The model under review builds one solid part; all positions refer to its coordinate system, in mm. Coordinates: 2 decimals unless noted, no trailing zeros. Loops run counter-clockwise (first coordinate to the right, second up) from the corner with the lowest first, then second, coordinate; pieces in that order, holes last. Notation, with made-up numbers: M -20,17 L 39,17 A19 ccw 39,49 Z; hole C 25.25,-31.5 d4. An arc over 180 degrees is marked long. Use CSV: the item, a comma, the result in double quotes. Start each with the question number.
1. Add section B-B, the plane y = -1.5. Write out the cut boundary in (x, z) (3 decimals), then the cut area to 3 significant figures.
2. Add section C-C, the plane z = 4.75. Write out the cut boundary in (x, y).
3. For L1, parallel to X at y = -5.25, z = 7.5; L2, parallel to X at y = -0.25, z = 2.25; L3, parallel to X at y = -1.75, z = 7.5, list the stretches that pass through material, from the lowest coordinate up.
4. Add section D-D, the plane x = 9. Write out the cut boundary in (y, z).
5. Draft analysis for pull direction X (two halves, no side actions). For faces 1 (the cylindrical face through (-0.22, -5.14, 0.9)), 2 (the cylindrical face through (15.235, -3.042, 7.303)), 3 (the cylindrical face through (-17.6, -1.48, 13.29)), state which applies: +X half, -X half, draft (parallel to the pull), parting line (faces both ways), or undercut.
6. Clearance check with flat-ended pins moving along their axes: P1, Ø1, axis at y = -4.5, z = 1.5, coming from the +X side; P2, Ø3, axis at x = -13.5, z = 7.075, coming from the -Y side; P3, Ø2, axis at x = -14.5, y = -4.5, coming from the -Z side; P4, Ø1, axis at x = -4.5, y = -4, coming from the +Z side. State where each tip first meets the part, or that it passes through.
7. Add section A-A, the plane x = 13.5. Write out the cut boundary in (y, z) (3 decimals), then the cut area to 3 significant figures.
from build123d import *

# Parameters (mm, degrees)
ESBO_O1_W                = 37
ESBO_O1_H                = 6
RESSALTO_EXTRUS_O1_DEPTH = 14.15
ESBO_O2_R                = 3.96875
CORTE_EXTRUS_O1_DEPTH    = 25.051455257
ESBO_O3_R                = 1.75
CORTE_EXTRUS_O2_DEPTH    = 13
FILETE2_R                = 3
FILETE3_R                = 3


with BuildPart() as part:
    # Esboço1 → Ressalto-extrusão1 (new body)
    with BuildSketch(Plane.XY):
        with Locations((0, -3)):
            Rectangle(ESBO_O1_W, ESBO_O1_H)
    extrude(amount=RESSALTO_EXTRUS_O1_DEPTH)

    # Esboço2 → Corte-extrusão1 (cut, through all)
    with BuildSketch(Plane(origin=(0, 0, 0), x_dir=(-1, 0, 0), z_dir=(0, 0, -1))):
        with Locations((-6, 0)):
            Circle(ESBO_O2_R)
        with Locations((5.752883735, 0)):
            Circle(ESBO_O2_R)
    extrude(amount=-CORTE_EXTRUS_O1_DEPTH, mode=Mode.SUBTRACT)

    # Esboço3 → Corte-extrusão2 (cut)
    with BuildSketch(Plane.XZ.offset(6)):
        with Locations(Location((-13.5, 7.075, 0), (0, 0, 270))):
            Circle(ESBO_O3_R)
        with Locations(Location((13.5, 7.075, 0), (0, 0, 270))):
            Circle(ESBO_O3_R)
    extrude(amount=-CORTE_EXTRUS_O2_DEPTH, mode=Mode.SUBTRACT)

    # Filete2
    # the kernel refuses this fillet: 3 mm, written as the material it takes off along each edge
    with BuildSketch(Plane(origin=(-26, -6, 0), x_dir=(0, 1, 0), z_dir=(1, 0, 0))) as filete2_piece_1:
        with BuildLine():
            CenterArc((FILETE2_R, FILETE2_R), FILETE2_R, 180, 90)
            Line((0, FILETE2_R), (0, 0))
            Line((0, 0), (FILETE2_R, 0))
        make_face()
    extrude(amount=52, mode=Mode.SUBTRACT)
    with BuildSketch(Plane(origin=(-26, -6, 14.15), x_dir=(0, 1, 0), z_dir=(1, 0, 0))) as filete2_piece_2:
        with BuildLine():
            CenterArc((FILETE2_R, -FILETE2_R), FILETE2_R, 90, 90)
            Line((0, -FILETE2_R), (0, 0))
            Line((0, 0), (FILETE2_R, 0))
        make_face()
    extrude(amount=52, mode=Mode.SUBTRACT)
    with BuildSketch(Plane(origin=(-18.5, -6, -7.5), x_dir=(1, 0, 0), z_dir=(0, 0, 1)), Plane(origin=(18.5, -6, -7.5), x_dir=(0, 1, 0), z_dir=(0, 0, 1))) as filete2_piece_3:
        with BuildLine():
            CenterArc((FILETE2_R, FILETE2_R), FILETE2_R, 180, 90)
            Line((0, FILETE2_R), (0, 0))
            Line((0, 0), (FILETE2_R, 0))
        make_face()
    extrude(amount=29.15, mode=Mode.SUBTRACT)

    # Filete3
    # the kernel refuses this fillet: 3 mm, written as the material it takes off along each edge
    with BuildSketch(Plane(origin=(15.5, -3, 11.15), x_dir=(0, 0, 1), z_dir=(1, 0, 0))) as filete3_piece_1_section:
        Polygon((0, 0), (FILETE3_R, 0), (FILETE3_R, FILETE3_R), (0, FILETE3_R), align=None)
    filete3_piece_1 = extrude(amount=FILETE3_R, mode=Mode.PRIVATE)
    filete3_piece_1 = filete3_piece_1 - Plane(origin=(15.5, -3, 11.15), x_dir=(0, 0.7071067811865475, -0.7071067811865475), z_dir=(1, 0, 0)) * Sphere(FILETE3_R, mode=Mode.PRIVATE)
    add(filete3_piece_1, mode=Mode.SUBTRACT)
    with BuildSketch(Plane(origin=(15.5, -3, 3), x_dir=(1, 0, 0), z_dir=(0, 0, -1))) as filete3_piece_2_section:
        Polygon((0, 0), (FILETE3_R, 0), (FILETE3_R, FILETE3_R), (0, FILETE3_R), align=None)
    filete3_piece_2 = extrude(amount=FILETE3_R, mode=Mode.PRIVATE)
    filete3_piece_2 = filete3_piece_2 - Plane(origin=(15.5, -3, 3), x_dir=(-0.7071067811865472, 0.7071067811865477, 0), z_dir=(0, 0, -1)) * Sphere(FILETE3_R, mode=Mode.PRIVATE)
    add(filete3_piece_2, mode=Mode.SUBTRACT)
    with BuildSketch(Plane(origin=(-15.5, -3, 11.15), x_dir=(-1, 0, 0), z_dir=(0, 0, 1))) as filete3_piece_3_section:
        Polygon((0, 0), (FILETE3_R, 0), (FILETE3_R, FILETE3_R), (0, FILETE3_R), align=None)
    filete3_piece_3 = extrude(amount=FILETE3_R, mode=Mode.PRIVATE)
    filete3_piece_3 = filete3_piece_3 - Plane(origin=(-15.5, -3, 11.15), x_dir=(0.7071067811865472, 0.7071067811865477, 0), z_dir=(0, 0, 1)) * Sphere(FILETE3_R, mode=Mode.PRIVATE)
    add(filete3_piece_3, mode=Mode.SUBTRACT)
    with BuildSketch(Plane(origin=(-15.5, -3, 3), x_dir=(-1, 0, 0), z_dir=(0, 0, -1))) as filete3_piece_4_section:
        Polygon((0, 0), (FILETE3_R, 0), (FILETE3_R, -FILETE3_R), (0, -FILETE3_R), align=None)
    filete3_piece_4 = extrude(amount=FILETE3_R, mode=Mode.PRIVATE)
    filete3_piece_4 = filete3_piece_4 - Plane(origin=(-15.5, -3, 3), x_dir=(0.7071067811865472, 0.7071067811865477, 0), z_dir=(0, 0, -1)) * Sphere(FILETE3_R, mode=Mode.PRIVATE)
    add(filete3_piece_4, mode=Mode.SUBTRACT)
    with BuildSketch(Plane(origin=(18.5, -3, 14.15), x_dir=(0, 0, -1), z_dir=(0, 1, 0)), Plane(origin=(-18.5, 7.5, 0), x_dir=(1, 0, 0), z_dir=(0, -1, 0)), Plane(origin=(18.5, -3, 0), x_dir=(-1, 0, 0), z_dir=(0, 1, 0))) as filete3_piece_5:
        with BuildLine():
            CenterArc((FILETE3_R, FILETE3_R), FILETE3_R, 180, 90)
            Line((0, FILETE3_R), (0, 0))
            Line((0, 0), (FILETE3_R, 0))
        make_face()
    extrude(amount=10.5, mode=Mode.SUBTRACT)
    with BuildSketch(Plane(origin=(-18.5, 7.5, 14.15), x_dir=(1, 0, 0), z_dir=(0, -1, 0))) as filete3_piece_6:
        with BuildLine():
            CenterArc((FILETE3_R, -FILETE3_R), FILETE3_R, 90, 90)
            Line((0, -FILETE3_R), (0, 0))
            Line((0, 0), (FILETE3_R, 0))
        make_face()
    extrude(amount=10.5, mode=Mode.SUBTRACT)


solid = part.part
Computed:
1,outline,"M -18.5,3 A3 ccw -15.5,0 L -9.427,0 L -9.427,14.15 L -15.5,14.15 A3 ccw -18.5,11.15 Z; M -2.079,0 L 2.326,0 L 2.326,14.15 L -2.079,14.15 Z; M 9.674,0 L 15.5,0 A3 ccw 18.5,3 L 18.5,11.15 A3 ccw 15.5,14.15 L 9.674,14.15 Z; hole C -13.5,7.075 d3.5; hole C 13.5,7.075 d3.5"
1,area,"289 mm^2"
2,outline,"M -18.5,-3 A3 ccw -15.5,-6 L 15.5,-6 A3 ccw 18.5,-3 L 18.5,0 L 9.97,0 A3.97 cw 2.03,0 L -1.78,0 A3.97 cw -9.72,0 L -18.5,0 Z"
3,L1,"x = -17.48 to -15.2, -11.8 to 11.8, 15.2 to 17.48"
3,L2,"x = -18.4 to -9.71, -1.79 to 2.04, 9.96 to 18.4"
3,L3,"x = -18.5 to -15.2, -11.8 to -9.31, -2.19 to 2.44, 9.56 to 11.8, 15.2 to 18.5"
4,outline,"M -6,3 A3 ccw -3,0 L -2.6,0 L -2.6,14.15 L -3,14.15 A3 ccw -6,11.15 Z"
5,face 1,"draft"
5,face 2,"undercut"
5,face 3,"-X half"
6,P1,"stops at x = 18.02"
6,P2,"passes through"
6,P3,"stops at z = 0.04"
6,P4,"stops at z = 14.08"
7,outline,"M -6,3 A3 ccw -3,0 L 0,0 L 0,5.325 L -6,5.325 Z; M -6,8.825 L 0,8.825 L 0,14.15 L -3,14.15 A3 ccw -6,11.15 Z"
7,area,"60.0 mm^2"
